The listing builds one solid part. Answer for the finished solid, in the listing's coordinates (mm). A direction names the side the tool comes from. Give positions to 0.01 mm unless a question says otherwise; leave off trailing zeros. Write each loop counter-clockwise with the first axis right and the second up, starting at its lowest first coordinate (ties: lowest second). Pieces come first, ordered by that corner, then holes. Notation, with made-up numbers: M 81,39 L 106,39 A25 ccw 106,66 Z; hole C 32,25.5 d3. An arc over 180 degrees is marked long. Answer as a JSON object with one key per item and string values.
```python
from build123d import *

# Parameters (mm, degrees)
SKETCH_1_W          = 80
SKETCH_1_H          = 60
SKETCH_1_R          = 1.6
EXTRUDE_1_DEPTH     = 50
SKETCH_2_W          = 76
SKETCH_2_H          = 58
CUT_EXTRUDE_1_DEPTH = 48
CUT_EXTRUDE_2_DEPTH = 81
FILLET_1_R          = 10


with BuildPart() as part:
    # 草图1 → 凸台-拉伸1 (new body)
    with BuildSketch(Plane.XY):
        with Locations((-8.993547962, 8.303805385)):
            Rectangle(SKETCH_1_W, SKETCH_1_H)
        with Locations((3.506452038, -1.696194615)):
            Circle(SKETCH_1_R, mode=Mode.SUBTRACT)
        with Locations((18.506452038, -1.696194615)):
            Circle(SKETCH_1_R, mode=Mode.SUBTRACT)
    extrude(amount=EXTRUDE_1_DEPTH)

    # 草图2 → 切除-拉伸1 (cut)
    with BuildSketch(Plane.XY.offset(50)):
        with Locations((-8.993547962, 7.303805385)):
            Rectangle(SKETCH_2_W, SKETCH_2_H)
    extrude(amount=-CUT_EXTRUDE_1_DEPTH, mode=Mode.SUBTRACT)

    # 草图3 → 切除-拉伸2 (cut, through all)
    with BuildSketch(Plane.ZY.offset(48.993547962)):
        Polygon((50, 30.864185465), (25, -21.696194615), (50, -21.696194615), align=None)
    extrude(amount=-CUT_EXTRUDE_2_DEPTH, mode=Mode.SUBTRACT)

    # 圆角1
    fillet_1_edges = [part.edges().sort_by_distance(p)[0] for p in [
        (-47.993547962, 30.864185465, 50),
        (30.006452038, 30.864185465, 50),
        (-47.993547962, -21.696194615, 25),
        (30.006452038, -21.696194615, 25),
    ]]
    fillet(fillet_1_edges, radius=FILLET_1_R)


solid = part.part
```
1. A cutting plane is placed at B-B, the plane z = 16. Give the vertices of the cut face in (x, y), plus the area to 3 significant figures.
Verdict:
{"outline": "M -48.99,-21.7 L -46.99,-21.7 L -46.99,36.3 L 29.01,36.3 L 29.01,-21.7 L 31.01,-21.7 L 31.01,38.3 L -48.99,38.3 Z", "area": "392 mm2"}
2. A cutting plane is placed at C-C, the plane y = 31.5. Give the vertices of the cut face in (x, z), plus the area to 3 significant figures.
Verdict:
{"outline": "M -48.99,0 L 31.01,0 L 31.01,49.87 L 29.01,49.87 L 29.01,2 L -46.99,2 L -46.99,49.87 L -48.99,49.87 Z", "area": "351 mm2"}
3. Consider line 1 along X through (y, z) = (-9, 18); line 2 along Y through (x, z) = (-9, 22); line 3 along Z through (x, y) = (-26.5, 5). Determine where each line is inside the solid, lowest interval first.
Verdict:
{"line 1": "x = -48.99 to -46.99, 29.01 to 31.01", "line 2": "y = 36.3 to 38.3", "line 3": "z = 0 to 2"}
4. A cutting plane is placed at D-D, the plane x = 3. Give the vertices of the cut face in (y, z), plus the area to 3 significant figures.
Verdict:
{"outline": "M -21.7,0 L -3.21,0 L -3.21,2 L -21.7,2 Z; M -0.18,0 L 38.3,0 L 38.3,50 L 36.3,50 L 36.3,2 L -0.18,2 Z", "area": "210 mm2"}
5. Flat-ended cylindrical pins translate along their axes: pin 1 (12 mm diameter, centred on x = -35, y = -10.5, fed in from +Z); pin 2 (3 mm diameter, centred on x = -24, z = 38.5, fed in from -Y). Find the tip coordinate at first contact, or state that the pin passes through.
Verdict:
{"pin 1": "stops at z = 2", "pin 2": "stops at y = 36.3"}
6. A cutting plane is placed at A-A, the plane x = -33.5. Give the vertices of the cut face in (y, z).
Verdict:
{"outline": "M -21.7,0 L 38.3,0 L 38.3,50 L 36.3,50 L 36.3,2 L -21.7,2 Z"}
7. For faces 1 (the flat face through (29.006, 13, 21)), 2 (the flat face through (29.99, 6.73, 38.52)), determine the directions among +Z, -Z, +X, -X, +Y, -Y from which every point of the face is accessible in a straight line to the end or side of a thin tool.
Verdict:
{"face 1": "+Z, -Y", "face 2": "+Z, +X, -X, -Y"}
8. The mould has two halves that part along Y. Classify faces 3 (the flat face through (-10, 38.304, 25)), 4 (the cylindrical face through (1.908, -1.626, 0.986)), 5 (the flat face through (-10, 37, 50)), 6 (the cylindrical face through (20.033, -1.216, 0.986)): released by +Y, released by -Y, zero draft, split by the parting line, or undercut.
Verdict:
{"face 3": "released by +Y", "face 4": "undercut", "face 5": "zero draft", "face 6": "undercut"}
